Can you work these out from the model? Positions are in its coordinate system, mm. A direction names the side the tool comes from. Round coordinates to 2 decimals unless told otherwise and drop trailing zeros. Loops run counter-clockwise (first coordinate to the right, second up) from the corner with the lowest first, then second, coordinate; pieces in that order, holes last. Notation, with made-up numbers: M 61,56.5 L 94,56.5 A22 ccw 94,85.5 Z; hole C 56.25,-22.75 d4. An arc over 180 degrees is marked long. Return JSON: item names as keys, results as strings.
```python
from build123d import *

# Parameters (mm, degrees)
SKETCH1_W           = 60
SKETCH1_H           = 80
BOSS_EXTRUDE1_DEPTH = 25
FILLET1_R           = 20
SKETCH3_R           = 7.95
CUT_EXTRUDE2_DEPTH  = 35
SKETCH5_W           = 60
SKETCH5_H           = 25
BOSS_EXTRUDE2_DEPTH = 3
SKETCH6_R           = 5
SKETCH6_R_2         = 1
CUT_EXTRUDE3_DEPTH  = 26
SKETCH7_R           = 2.5
CUT_EXTRUDE4_DEPTH  = 15
SKETCH8_W           = 0.5
SKETCH8_H           = 1.458969306
SKETCH8_H_2         = 7.530561822
CUT_EXTRUDE5_DEPTH  = 26


with BuildPart() as part:
    # Sketch1 → Boss-Extrude1 (new body)
    with BuildSketch(Plane(origin=(0, 0, 0), x_dir=(1, 0, 0), z_dir=(0, 1, 0))):
        Rectangle(SKETCH1_W, SKETCH1_H)
    extrude(amount=BOSS_EXTRUDE1_DEPTH)

    # Fillet1
    fillet1_edges = [part.edges().sort_by_distance(p)[0] for p in [
        (-30, 12.5, -40),
        (30, 12.5, -40),
    ]]
    fillet(fillet1_edges, radius=FILLET1_R)

    # Sketch3 → Cut-Extrude2 (cut)
    with BuildSketch(Plane(origin=(0, 25, 0), x_dir=(1, 0, 0), z_dir=(0, 1, 0))):
        with Locations((-20.9, -29.964854959)):
            Circle(SKETCH3_R)
        with Locations((20.9, -29.964854959)):
            Circle(SKETCH3_R)
    extrude(amount=-CUT_EXTRUDE2_DEPTH, mode=Mode.SUBTRACT)

    # Sketch5 → Boss-Extrude2 (add)
    with BuildSketch(Plane.XY.offset(40)):
        with Locations((0, 12.5)):
            Rectangle(SKETCH5_W, SKETCH5_H)
    extrude(amount=BOSS_EXTRUDE2_DEPTH)

    # Sketch6 → Cut-Extrude3 (cut, through all)
    with BuildSketch(Plane(origin=(0, 25, 0), x_dir=(1, 0, 0), z_dir=(0, 1, 0))):
        with Locations((0, -29.964854959)):
            Circle(SKETCH6_R)
        with Locations((0, -37.964854959)):
            Circle(SKETCH6_R_2)
        with Locations((8, -29.964854959)):
            Circle(SKETCH6_R_2)
        with Locations((0, -21.964854959)):
            Circle(SKETCH6_R_2)
        with Locations((-8, -29.964854959)):
            Circle(SKETCH6_R_2)
    extrude(amount=-CUT_EXTRUDE3_DEPTH, mode=Mode.SUBTRACT)

    # Sketch7 → Cut-Extrude4 (cut)
    with BuildSketch(Plane(origin=(0, 0, 0), x_dir=(-1, 0, 0), z_dir=(0, -1, 0))):
        with Locations((-0.26141162, 23.519285142)):
            Circle(SKETCH7_R)
    extrude(amount=-CUT_EXTRUDE4_DEPTH, mode=Mode.SUBTRACT)

    # Sketch8 → Cut-Extrude5 (cut, through all)
    with BuildSketch(Plane.XZ):
        with BuildLine():
            ThreePointArc((20.828077187, 37.914529614), (21.078165346, 37.9128583), (21.328077187, 37.903321431))
            Line((21.328077187, 37.903321431), (21.328077187, 43))
            Line((21.328077187, 43), (20.828077187, 43))
            Line((20.828077187, 43), (20.828077187, 37.914529614))
        make_face()
        with Locations((21.078077187, 43.729484653)):
            Rectangle(SKETCH8_W, SKETCH8_H)
        with BuildLine():
            Line((21.328077187, 37.903321431), (21.328077187, 36.928407484))
            Line((21.328077187, 36.928407484), (20.828077187, 36.928407484))
            Line((20.828077187, 36.928407484), (20.828077187, 37.914529614))
            ThreePointArc((20.828077187, 37.914529614), (15.303987418, 24.317984748), (28.85, 29.964854959))
            ThreePointArc((28.85, 29.964854959), (26.670862745, 35.432911578), (21.328077187, 37.903321431))
        make_face()
        with BuildLine():
            Line((20.828077187, 36.928407484), (21.328077187, 36.928407484))
            Line((21.328077187, 36.928407484), (21.328077187, 37.903321431))
            ThreePointArc((21.328077187, 37.903321431), (21.078165346, 37.9128583), (20.828077187, 37.914529614))
            Line((20.828077187, 37.914529614), (20.828077187, 36.928407484))
        make_face()
        with Locations((-20.848704866, 40.693688395)):
            Rectangle(SKETCH8_W, SKETCH8_H_2)
    extrude(amount=-CUT_EXTRUDE5_DEPTH, mode=Mode.SUBTRACT)


solid = part.part
```
Q1. Suppose I cut it at C-C, the plane y = 23.75. Please give me the cut outline in (x, z).
Results:
{"outline": "M -30,-20 A20 ccw -10,-40 L 10,-40 A20 ccw 30,-20 L 30,43 L 21.33,43 L 21.33,37.9 A7.95 cw long 20.83,37.91 L 20.83,43 L -20.6,43 L -20.6,37.91 A7.95 cw long -21.1,37.91 L -21.1,43 L -30,43 Z; hole C -8,29.96 d2; hole C 0,29.96 d10; hole C 0,21.96 d2; hole C 0,37.96 d2; hole C 8,29.96 d2"}
Q2. I'm going to push flat-ended pins straight in: pin 1 Ø3 at (x, z) = (0.26, -23.52) entering from -Y; pin 2 Ø1 at (x, y) = (13.5, 17) entering from -Z. Where does each tip first touch, or does it pass through?
Results:
{"pin 1": "stops at y = 15", "pin 2": "stops at z = -39.77"}
Q3. Suppose I cut it at D-D, the plane z = -22. Please give me the cut outline in (x, y).
Results:
{"outline": "M -29.9,0 L -1.72,0 L -1.72,15 L 2.25,15 L 2.25,0 L 29.9,0 L 29.9,25 L -29.9,25 Z"}
Q4. Thinking about a two-plate mould opening in X: for faces 1 (the flat face through (-26, 13, 43)), 2 (the cylindrical face through (-24.297, 12.675, -33.986)), 3 (the flat face through (-21.099, 12, 40)), 4 (the cylindrical face through (-0.651, 12.675, 25.007)), which applies, pulls with the +X half, pulls with the -X half, needs draft (parallel to the pull), parting line crosses it, or undercut?
Results:
{"face 1": "needs draft", "face 2": "pulls with the -X half", "face 3": "undercut", "face 4": "undercut"}
Q5. Suppose I cut it at A-A, the plane x = -8. Please give me the cut outline in (y, z).
Results:
{"outline": "M 0,-40 L 25,-40 L 25,28.96 L 0,28.96 Z; M 0,30.96 L 25,30.96 L 25,43 L 0,43 Z"}
Q6. If I drill on line 1 along Z through (x, y) = (0, 15.25); line 2 along Z through (x, y) = (0, 12.25); line 3 along X through (y, z) = (18, 23), over which ranges is the centre line in solid material (lowest first)?
Results:
{"line 1": "z = -40 to 20.96, 22.96 to 24.96, 34.96 to 36.96, 38.96 to 43", "line 2": "z = -40 to -26.01, -21.03 to 20.96, 22.96 to 24.96, 34.96 to 36.96, 38.96 to 43", "line 3": "x = -30 to -24.73, -17.07 to 17.07, 24.73 to 30"}
Q7. Suppose I cut it at B-B, the plane y = 1.5. Please give me the cut outline in (x, z).
Results:
{"outline": "M -30,-20 A20 ccw -10,-40 L 10,-40 A20 ccw 30,-20 L 30,43 L 21.33,43 L 21.33,37.9 A7.95 cw long 20.83,37.91 L 20.83,43 L -20.6,43 L -20.6,37.91 A7.95 cw long -21.1,37.91 L -21.1,43 L -30,43 Z; hole C -8,29.96 d2; hole C 0,29.96 d10; hole C 0.26,-23.52 d5; hole C 0,21.96 d2; hole C 0,37.96 d2; hole C 8,29.96 d2"}
Q8. On a 3-axis mill with a long thin cutter (end or side, diameter ignored), from which of +Z, -Z, +X, -X, +Y, -Y can I reach the whole of each face in a straight line? I mean faces 5 (the flat face through (0, 15, -24)), 6 (the flat face through (21.328, 12, 40)), 7 (the flat face through (26, 13, 43)). Say none if no direction works.
Results:
{"face 5": "-Y", "face 6": "+Z, +Y, -Y", "face 7": "+Z, +X, -X, +Y, -Y"}
